Check sheet for the modelled part. Datum: model origin and axes. Units: mm. Face numbers are marked on the shaded views. Round coordinates to 2 decimals unless told otherwise and drop trailing zeros. Loops run counter-clockwise (first coordinate to the right, second up) from the corner with the lowest first, then second, coordinate; pieces in that order, holes last. Notation, with made-up numbers: (-5, 18) - (10, 18) arc R8 cw to (10, 33) - close; hole circle Ø1 at (-37, -15.75). An arc over 180 degrees is marked (long way). Answer in a Markdown table with one row per item. Add a question column.
(1) Gauge pin test, flat ends, axial feed: pin 1 (1.6 mm diameter, centred on x = -2, z = -57, fed in from +Y); pin 2 (1.2 mm diameter, centred on y = 1.5, z = -33, fed in from +X); pin 3 (2 mm diameter, centred on x = -31, z = -23.3, fed in from -Y); pin 4 (0.5 mm diameter, centred on y = 14, z = -59, fed in from +X). Record the tip position at first contact, or that the pin passes through.
(2) Cross-section at B-B on z = -30. Enter the section's corners in (x, y), then the cut area to 3 significant figures.
(3) Thickness scan on line 1 along Z through (x, y) = (-3, 1.45); line 2 along X through (y, z) = (2.55, -23.3); line 3 along Z through (x, y) = (-20, 0.75). Record the ranges inside material, lowest first.
(4) Cross-section at C-C on y = 3.25. Count the separate pieces of the cut face and the enclosed holes in it, then the cut area to 3 significant figures.
(5) Mould release check, pull along X, two halves, no side actions. Record for the marked faces 1 and 2: +X half, -X half, draft (parallel to the pull), parting line (faces both ways), or undercut.
(6) Cross-section at D-D on y = 10.5. Enter the section's corners in (x, z).
(7) Cross-section at A-A on x = -20. Enter the section's corners in (y, z).
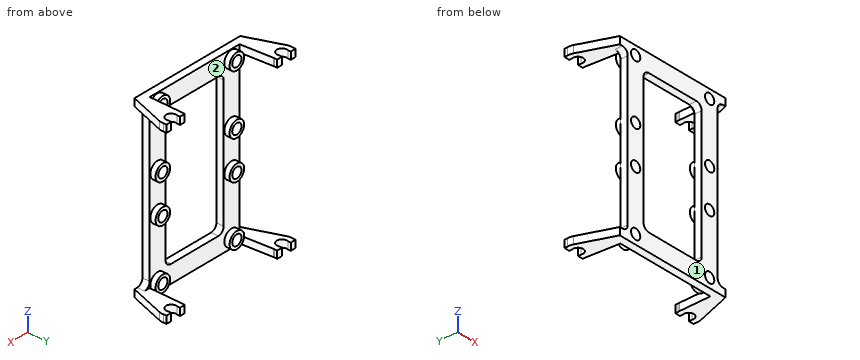
Autodesk Inventor part; units mm, degrees
ref_plane "YZ Plane" through (0, 0, 0) normal (1, 0, 0) x (0, 1, 0)
ref_plane "XZ Plane" through (0, 0, 0) normal (0, 1, 0) x (-1, 0, 0)
ref_plane "XY Plane" through (0, 0, 0) normal (0, 0, 1) x (1, 0, 0)
sketch "Sketch1" plane through (0, 0, 0) normal (0, 1, 0) x (-1, 0, 0)
  line L0 (0, 0) -> (34, 0)
  line L1 (34, 0) -> (34, -60)
  line L2 (34, -60) -> (0, -60)
  line L3 (0, -60) -> (0, 0)
  dimension "d0" = 34
  dimension "d1" = 60
extrude "Extrusion1" add sketch "Sketch1" along normal blind 2.5
sketch "Sketch4" plane through (-34, 0, 0) normal (0, 0, 1) x (1, 0, 0)
  circle A0 centre (-4.5, 13) radius 1.75
  circle A1 centre (-4.5, 13) radius 3.5
  circle A2 centre (37.41, 13) radius 1.75
  circle A3 centre (37.41, 13) radius 3.5
  line L0 (0, 0) -> (0, 2.5)
  line L1 (0, 2.5) -> (34, 2.5)
  line L2 (0, 2.5) -> (-1.0153, 13.3268)
  line L3 (34, 0) -> (0, 0)
  line L4 (0, 0) -> (-3, 0)
  line L5 (-3, 0) -> (-7.743, 11.6835)
  line L6 (34, 2.5) -> (33.9101, 12.97)
  line L7 (34, 0) -> (37, 0)
  line L8 (37, 0) -> (40.7495, 11.9524)
  line L9 (34, 0) -> (34, 2.5)
  line L10 (34, 2.5) -> (34, 0)
  dimension "d4" = 3.5
  dimension "d5" = 7
  dimension "d6" = 4.5
  dimension "d7" = 41.91
  dimension "d8" = 10.5
  dimension "d9" = 3
  dimension "d10" = 3
extrude "Extrusion2" add sketch "Sketch4" against normal blind 2.5 contours A1 | A1 L2 L0 L4 L5 | L6 A3 L8 L7 L9 | A3
pattern_linear "Rectangular Pattern1" count 2 spacing 57.5 along (0, 0, -1) of "Extrusion2"
hole "Hole1" at (-31, 2.5, -3) direction (0, -1, 0) diameter 3.5 end through all
sketch "Sketch7" plane through (0, 2.5, 0) normal (0, 1, 0) x (1, 0, 0)
  circle A0 centre (-31, 3) radius 1.75
  circle A1 centre (-31, 3) radius 2.75
  point P0 (0, 0)
  dimension "d37" = 5.5
extrude "Extrusion3" add sketch "Sketch7" along normal blind 1.8
pattern_linear "Rectangular Pattern2" count 2 spacing 28 along (1, 0, 0) count 2 spacing 20.3 along (0, 0, -1) of "Hole1", "Extrusion3"
pattern_linear "Rectangular Pattern3" count 2 spacing 33.5 along (0, 0, -1) of "Rectangular Pattern2", "Extrusion3", "Hole1"
sketch "Sketch8" plane through (0, 2.5, 0) normal (0, 1, 0) x (1, 0, 0)
  circle A0 centre (-3, 56.8) radius 2.75
  circle A1 centre (-31, 56.8) radius 2.75
  circle A2 centre (-3, 36.5) radius 2.75
  circle A3 centre (-31, 36.5) radius 2.75
  circle A4 centre (-3, 23.3) radius 2.75
  circle A5 centre (-31, 23.3) radius 2.75
  circle A6 centre (-3, 3) radius 2.75
  circle A7 centre (-31, 3) radius 2.75
  line L0 (-34, 0) -> (0, 0)
  line L1 (0, 0) -> (0, 2.5)
  line L2 (0, 2.5) -> (0, 57.5)
  line L3 (0, 57.5) -> (0, 60)
  line L4 (0, 60) -> (-34, 60)
  line L5 (-34, 60) -> (-34, 57.5)
  line L6 (-34, 57.5) -> (-34, 2.5)
  line L7 (-34, 2.5) -> (-34, 0)
  line L8 (-28, 6) -> (-28, 54)
  line L9 (-28, 54) -> (-6, 54)
  line L10 (-6, 54) -> (-6, 6)
  line L11 (-6, 6) -> (-28, 6)
  dimension "d48" = 6
extrude "Extrusion4" cut sketch "Sketch8" against normal through all contours L8 L9 L10 L11
fillet "Fillet1" radius 2 8 edges at (-34, 1.25, -2.5) (-34, 1.25, -57.5) (0, 1.25, -57.5) (0, 1.25, -2.5) (-6, 1.25, -6) (-28, 1.25, -6) (-28, 1.25, -54) (-6, 1.25, -54)
sketch "Sketch9" plane through (-37, 0, 0) normal (0, 0, 1) x (1, 0, 0)
  circle A0 centre (-1.5, 13) radius 1.75 construction
  line L0 (-7.7139, 20.5221) -> (44.4141, 20.5221)
  line L1 (44.4141, 20.5221) -> (44.4141, 13.5)
  line L2 (44.4141, 13.5) -> (-7.7139, 13.5)
  line L3 (-7.7139, 13.5) -> (-7.7139, 20.5221)
  point P0 (37, 0)
extrude "Extrusion5" cut sketch "Sketch9" against normal through all
sketch "Sketch11" plane through (-36.8229, 13.5, 0) normal (0, 1, 0) x (1, 0, 0)
  line L0 (-3.3541, 2.5) -> (-3.3541, 0)
  line L1 (-5.1412, 2.5) -> (-3.3541, 2.5)
  line L2 (-5.1412, 0) -> (-5.1412, 2.5)
  line L3 (-3.3541, 0) -> (-5.1412, 0)
  line L4 (0, 0) -> (0, 2.5)
  line L5 (1.7871, 0) -> (0, 0)
  line L6 (1.7871, 2.5) -> (1.7871, 0)
  line L7 (0, 2.5) -> (1.7871, 2.5)
  line L8 (-3.3541, 57.5) -> (-5.1412, 57.5)
  line L9 (-3.3541, 60) -> (-3.3541, 57.5)
  line L10 (-5.1412, 60) -> (-3.3541, 60)
  line L11 (-5.1412, 57.5) -> (-5.1412, 60)
  line L12 (1.7871, 57.5) -> (0, 57.5)
  line L13 (1.7871, 60) -> (1.7871, 57.5)
  line L14 (0, 60) -> (1.7871, 60)
  line L15 (0, 57.5) -> (0, 60)
  line L16 (36.7688, 57.5) -> (36.7688, 60)
  line L17 (38.5559, 57.5) -> (36.7688, 57.5)
  line L18 (38.5559, 60) -> (38.5559, 57.5)
  line L19 (36.7688, 60) -> (38.5559, 60)
  line L20 (43.6971, 60) -> (43.6971, 57.5)
  line L21 (41.91, 60) -> (43.6971, 60)
  line L22 (41.91, 57.5) -> (41.91, 60)
  line L23 (43.6971, 57.5) -> (41.91, 57.5)
  line L24 (36.7688, 0) -> (36.7688, 2.5)
  line L25 (38.5559, 0) -> (36.7688, 0)
  line L26 (38.5559, 2.5) -> (38.5559, 0)
  line L27 (36.7688, 2.5) -> (38.5559, 2.5)
  line L28 (43.6971, 2.5) -> (43.6971, 0)
  line L29 (41.91, 2.5) -> (43.6971, 2.5)
  line L30 (41.91, 0) -> (41.91, 2.5)
  line L31 (43.6971, 0) -> (41.91, 0)
  point P0 (36.8229, 0)
extrude "Extrusion7" add sketch "Sketch11" along normal blind 1
properties part number "RelayHolderREV2" material "ABS Plastic"
Answers:
| question | item | result |
|---|---|---|
| 1 | pin 1 | stops at y = 4.3 |
| 1 | pin 2 | stops at x = 0 |
| 1 | pin 3 | passes through |
| 1 | pin 4 | stops at x = 6.87 |
| 2 | outline | (-34, 0) - (-28, 0) - (-28, 2.5) - (-34, 2.5) - close; (-6, 0) - (0, 0) - (0, 2.5) - (-6, 2.5) - close |
| 2 | area | 30.0 mm^2 |
| 3 | line 1 | z = -60 to -58.55, -55.05 to -38.25, -34.75 to -25.05, -21.55 to -4.75, -1.25 to 0 |
| 3 | line 2 | x = -33.75 to -32.75, -29.25 to -28.25, -5.75 to -4.75, -1.25 to -0.25 |
| 3 | line 3 | z = -60 to -54, -6 to 0 |
| 4 | separate pieces | 12 |
| 4 | enclosed holes | 8 |
| 4 | area | 154 mm^2 |
| 5 | face 1 | draft |
| 5 | face 2 | undercut |
| 6 | outline | (-41.26, -60) - (-34.75, -60) - (-34.75, -57.5) - (-41.26, -57.5) - close; (-41.26, -2.5) - (-34.75, -2.5) - (-34.75, 0) - (-41.26, 0) - close; (-0.07, -60) - (6.29, -60) - (6.29, -57.5) - (-0.07, -57.5) - close; (-0.07, -2.5) - (6.29, -2.5) - (6.29, 0) - (-0.07, 0) - close |
| 7 | outline | (0, -60) - (2.5, -60) - (2.5, -54) - (0, -54) - close; (0, -6) - (2.5, -6) - (2.5, 0) - (0, 0) - close |
